Verification items for the finished model (mm, model axes). Face numbers are marked on the shaded views. A direction names the side the tool comes from. Give positions to 0.01 mm unless a question says otherwise; leave off trailing zeros. Loops run counter-clockwise (first coordinate to the right, second up) from the corner with the lowest first, then second, coordinate; pieces in that order, holes last. Notation, with made-up numbers: M 76.25,7.25 L 83.25,7.25 A18 ccw 83.25,16.25 Z; hole C -12.75,-37.75 d5. An arc over 180 degrees is marked long. Use CSV: the item, a comma, the result in double quotes.
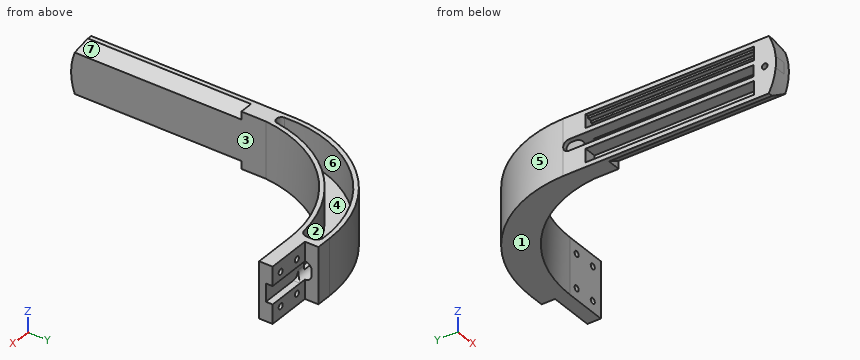
from build123d import *
from OCP.BRepAlgoAPI import BRepAlgoAPI_Cut
from OCP.TopTools import TopTools_ListOfShape

# Parameters (mm, degrees)
EXTRUDE_1_DEPTH      = 25
SKETCH_2_W           = 20
SKETCH_2_H           = 6
CUT_EXTRUDE_1_DEPTH  = 174.245490562
CUT_EXTRUDE_2_DEPTH  = 76
CUT_EXTRUDE_4_DEPTH  = 5
CUT_EXTRUDE_3_REACH  = 175.245
FILLET_3_R           = 2
FILLET_4_R           = 3
CUT_EXTRUDE_6_DEPTH  = 75
M3X0_51_D            = 2.5
CUT_EXTRUDE_7_REACH  = 175.245
SKETCH_13_W          = 20
SKETCH_13_H          = 8
CUT_EXTRUDE_8_DEPTH  = 3
FILLET_8_R           = 3
CUT_EXTRUDE_9_DEPTH  = 28
CUT_EXTRUDE_10_DEPTH = 6
EXTRUDE_2_DEPTH      = 5
M3X0_52_D            = 2.5
M3X0_52_DEPTH        = 4
M3X0_52_TIP          = 0.751075774


with BuildPart() as part:
    # Эскиз1 → Бобышка-Вытянуть1 (new body)
    with BuildSketch(Plane.XY):
        with BuildLine():
            Line((0, 0), (0, 95))
            ThreePointArc((0, 95), (16.753981094, 133.950491977), (56, 150))
            Line((56, 150), (83, 150))
            Line((83, 150), (83, 138))
            Line((83, 138), (64, 138))
            ThreePointArc((64, 138), (26.128506763, 123.339286692), (8, 87))
            Line((8, 87), (8, 0))
            Line((8, 0), (0, 0))
        make_face()
    extrude(amount=EXTRUDE_1_DEPTH)

    # Эскиз2 → Вырез-Вытянуть1 (cut, through all)
    with BuildSketch(Plane.XY.offset(25)):
        with Locations((73, 147)):
            Rectangle(SKETCH_2_W, SKETCH_2_H)
    extrude(amount=-CUT_EXTRUDE_1_DEPTH, mode=Mode.SUBTRACT)

    # Эскиз5 → Вырез-Вытянуть2 (cut)
    with BuildSketch(Plane.XZ):
        Polygon((8, 3.464101615), (2, 0), (8, 0), align=None)
        Polygon((8, 25), (8, 21.535898385), (2, 25), align=None)
    extrude(amount=-CUT_EXTRUDE_2_DEPTH, mode=Mode.SUBTRACT)

    # Эскиз6 → Вырез-Вытянуть4 (cut)
    with BuildSketch(Plane.ZY):
        with BuildLine():
            Line((10, -11.91606518), (10, 92.5))
            ThreePointArc((10, 92.5), (12.5, 95), (15, 92.5))
            Line((15, 92.5), (15, -11.91606518))
            ThreePointArc((15, -11.91606518), (12.5, -14.41606518), (10, -11.91606518))
        make_face()
    extrude(amount=-CUT_EXTRUDE_4_DEPTH, mode=Mode.SUBTRACT)

    # Вырез-Вытянуть3: up to this face of the body (flat: up to its plane)
    cut_extrude_3_end = Plane(part.part.faces().sort_by_distance((2.5, 46.25, 10))[0])
    # Эскиз3 → Вырез-Вытянуть3 (cut, up to the picked face)
    with BuildSketch(Plane(origin=(0, 0, 25), x_dir=(-1, 0, 0), z_dir=(0, 0, -1)), mode=Mode.PRIVATE) as cut_extrude_3_sk1:
        with BuildLine():
            Line((-60, 147.851673111), (-60, 139.862487056))
            ThreePointArc((-60, 139.862487056), (-24.008081752, 124.100361226), (-6.215777406, 89.067566648))
            Line((-6.215777406, 89.067566648), (-2.215777406, 89.067566648))
            ThreePointArc((-2.215777406, 89.067566648), (-17.483639866, 131.852128074), (-60, 147.851673111))
        make_face()
    cut_extrude_3_tool1 = split(extrude(cut_extrude_3_sk1.sketch, amount=CUT_EXTRUDE_3_REACH, mode=Mode.PRIVATE), bisect_by=cut_extrude_3_end, keep=Keep.BOTH, mode=Mode.PRIVATE)
    add(cut_extrude_3_tool1.solids().sort_by(Axis((26.403402, 126.933471, 25), (0, 0, -1)))[0], mode=Mode.SUBTRACT)

    # Скругление3
    fillet_3_edges = [part.edges().sort_by_distance(p)[0] for p in [
        (6.215777406, 89.067566648, 17.5),
        (2.215777406, 89.067566648, 20),
    ]]
    fillet(fillet_3_edges, radius=FILLET_3_R)

    # Скругление4
    fillet_4_edges = [part.edges().sort_by_distance(p)[0] for p in [
        (60, 139.862487056, 17.5),
        (60, 147.851673111, 17.5),
    ]]
    fillet(fillet_4_edges, radius=FILLET_4_R)

    # Эскиз8 → Вырез-Вытянуть6 (cut)
    with BuildSketch(Plane(origin=(0, 10, 0), x_dir=(1, 0, 0), z_dir=(0, 1, 0))):
        Polygon((0, -2), (1.5, -2), (1.5, -3), (3.5, -3), (3.5, -4), (5.5, -4), (5.5, -8), (0, -8), align=None)
        Polygon((3.5, -22), (3.5, -21), (5.5, -21), (5.5, -17), (0, -17), (0, -23), (1.5, -23), (1.5, -22), align=None)
    extrude(amount=CUT_EXTRUDE_6_DEPTH, mode=Mode.SUBTRACT)

    # Отверстие обработанное метчиком M3x0.51 (through all)
    with Locations(Plane(origin=(19.191951444, 144, 18.799685968), x_dir=(1, 0, 0), z_dir=(0, 1, 0))):
        with Locations((48.808048556, 13.799685968), (58.808048556, 13.799685968), (58.808048556, -1.200314032), (48.808048556, -1.200314032)):
            Hole(M3X0_51_D / 2)

    # Эскиз12 → Вырез-Вытянуть7 (cut, up to next)
    with BuildSketch(Plane.ZY, mode=Mode.PRIVATE) as cut_extrude_7_sk1:
        with BuildLine():
            Line((0, 3.30197377), (0, 0))
            Line((0, 0), (12.5, 0))
            Line((12.5, 0), (25, 0))
            Line((25, 0), (25, 3.30197377))
            ThreePointArc((25, 3.30197377), (12.5, 0.1), (0, 3.30197377))
        make_face()
    cut_extrude_7_tool1 = extrude(cut_extrude_7_sk1.sketch, amount=-CUT_EXTRUDE_7_REACH, mode=Mode.PRIVATE) & part.part
    add(cut_extrude_7_tool1.solids().sort_by_distance((0, 1.650987, 0.252171))[0], mode=Mode.SUBTRACT)

    # Эскиз13 → Вырез-Вытянуть8 (cut)
    with BuildSketch(Plane(origin=(0, 144, 0), x_dir=(1, 0, 0), z_dir=(0, 1, 0))):
        with Locations((73, -12.5)):
            Rectangle(SKETCH_13_W, SKETCH_13_H)
    extrude(amount=-CUT_EXTRUDE_8_DEPTH, mode=Mode.SUBTRACT)

    # Скругление8
    fillet_8_edges = [part.edges().sort_by_distance(p)[0] for p in [
        (63, 142.5, 16.5),
        (63, 142.5, 8.5),
    ]]
    fillet(fillet_8_edges, radius=FILLET_8_R)


with BuildPart() as cut_extrude_9_tool:
    # Эскиз14 → Вырез-Вытянуть9 (new body)
    with BuildSketch(Plane(origin=(83, 0, 0), x_dir=(0, 0, -1), z_dir=(1, 0, 0))):
        with BuildLine():
            Line((-13.5, 147), (-11.5, 147))
            ThreePointArc((-11.5, 147), (-8.5, 144), (-11.5, 141))
            Line((-11.5, 141), (-13.5, 141))
            ThreePointArc((-13.5, 141), (-16.5, 144), (-13.5, 147))
        make_face()
    extrude(amount=-CUT_EXTRUDE_9_DEPTH)


with BuildPart() as part_1:
    add(part.part)

    # Вырез-Вытянуть9: cut by cut_extrude_9_tool, with a tolerance
    cut_extrude_9_stock = TopTools_ListOfShape()
    cut_extrude_9_stock.Append(part_1.part.wrapped)
    cut_extrude_9_tools = TopTools_ListOfShape()
    cut_extrude_9_tools.Append(cut_extrude_9_tool.part.wrapped)
    cut_extrude_9_cut = BRepAlgoAPI_Cut()
    cut_extrude_9_cut.SetArguments(cut_extrude_9_stock)
    cut_extrude_9_cut.SetTools(cut_extrude_9_tools)
    cut_extrude_9_cut.SetFuzzyValue(0.00001)
    cut_extrude_9_cut.Build()
    add(Compound.cast(cut_extrude_9_cut.Shape()).solids(), mode=Mode.REPLACE)

    # Эскиз15 → Вырез-Вытянуть10 (cut)
    with BuildSketch(Plane.ZY):
        with BuildLine():
            Line((15, 92.5), (15, 85.5))
            ThreePointArc((15, 85.5), (12.5, 83), (10, 85.5))
            Line((10, 85.5), (10, 92.5))
            ThreePointArc((10, 92.5), (12.5, 95), (15, 92.5))
        make_face()
    extrude(amount=-CUT_EXTRUDE_10_DEPTH, mode=Mode.SUBTRACT)

    # Эскиз19 → Бобышка-Вытянуть2 (add)
    with BuildSketch(Plane.ZY):
        with BuildLine():
            Line((10, 10.1), (10, 0.220471411))
            ThreePointArc((10, 0.220471411), (12.5, 0.1), (15, 0.220471411))
            Line((15, 0.220471411), (15, 10.1))
            Line((15, 10.1), (10, 10.1))
        make_face()
    extrude(amount=-EXTRUDE_2_DEPTH)

    # Отверстие обработанное метчиком M3x0.52
    with Locations(Plane.ZY):
        with Locations((12.5, 5.1)):
            Hole(M3X0_52_D / 2, depth=M3X0_52_DEPTH)
            with Locations((0, 0, -(M3X0_52_DEPTH + M3X0_52_TIP / 2))):  # 118° drill point
                Cone(0, M3X0_52_D / 2, M3X0_52_TIP, mode=Mode.SUBTRACT)


solid = part_1.part
(1) Scan lines: L1, parallel to Z at x = 78, y = 140.9; L2, parallel to Z at x = 78, y = 142; L3, parallel to X at y = 140.85, z = 5. Record each from-to range of solid material in increasing order. Write a range as from..to.
Calculated:
L1,"z = 0..3.75, 6.25..18.75, 21.25..25"
L2,"z = 0..3.75, 6.25..8.5, 16.5..18.75, 21.25..25"
L3,"x = 25.32..66.75, 69.25..76.75, 79.25..83"
(2) Mould release check, pull along Y, two halves, no side actions. Record for the marked faces 5, 6 and 7: released by +Y, released by -Y, zero draft, split by the parting line, or undercut.
Calculated:
face 5,"released by +Y"
face 6,"undercut"
face 7,"zero draft"
(3) Depth check by flat-ended pin: pin 1 Ø5 at (x, z) = (44, 16.5) entering from -Y; pin 2 Ø12 at (y, z) = (74.5, 14) entering from +X; pin 3 Ø4 at (x, z) = (65, 6) entering from -Y. Enter the tip coordinate at first touch or a pass-through.
Calculated:
pin 1,"stops at y = 133.3"
pin 2,"stops at x = 8"
pin 3,"stops at y = 137.99"
(4) Section check A-A on y = 40. Record the cut outline in (x, z).
Calculated:
outline,"M 0,0 L 2,0 L 8,3.46 L 8,21.54 L 2,25 L 0,25 L 0,23 L 1.5,23 L 1.5,22 L 3.5,22 L 3.5,21 L 5.5,21 L 5.5,17 L 0,17 L 0,15 L 5,15 L 5,10 L 0,10 L 0,8 L 5.5,8 L 5.5,4 L 3.5,4 L 3.5,3 L 1.5,3 L 1.5,2 L 0,2 Z"
(5) Section check B-B on x = 24. Record the cut outline in (y, z), plus the area to 3 significant figures.
Calculated:
outline,"M 121.3,0 L 139.96,0 L 139.96,25 L 137.5,25 L 137.5,10 L 124.09,10 L 124.09,25 L 121.3,25 Z"
area,"265 mm²"
(6) Section check C-C on y = 98. Record the cut outline in (x, z), plus the area to 3 significant figures.
Calculated:
outline,"M 0.13,0 L 10.15,0 L 10.15,25 L 8.07,25 L 8.07,10 L 2.14,10 L 2.14,25 L 0.13,25 Z"
area,"162 mm²"
(7) Tool access check on the marked faces 1, 2, 3 and 4. Record the directions out of +Z, -Z, +X, -X, +Y, -Y that give a thin tool (end or side, any length) a straight path to the whole face; none if there is none.
Calculated:
face 1,"-Z, +X, -X, +Y, -Y"
face 2,"+Z"
face 3,"+Z, -Z, +X, -Y"
face 4,"none"
